```python
from build123d import *

# Parameters (mm, degrees)
F0_R     = 12.5
F1_DEPTH = 50
F2_SIZE  = 2
F3_R     = 8.107288
F4_DEPTH = 20
F5_W     = 25
F5_H     = 25
F6_DEPTH = 30
F7_SIZE  = 2.5
F8_R     = 10
F9_DEPTH = 50.001


with BuildPart() as f1:
    # F0 (on Top) → F1 (new body)
    with BuildSketch(Plane.XY):
        Circle(F0_R)
    extrude(amount=F1_DEPTH)

    # F2
    f2_edges = [f1.edges().sort_by_distance(p)[0] for p in [
        (-12.5, 0, 50),
        (-12.5, 0, 0),
    ]]
    chamfer(f2_edges, length=F2_SIZE)

    # F3 (on Front) → F4 (join)
    with BuildSketch(Plane.XZ):
        with Locations((0, 24.859188)):
            Circle(F3_R)
    extrude(amount=F4_DEPTH)

    # F5 (on face) → F6 (join)
    with BuildSketch(Plane.XZ.offset(20)):
        with Locations((0, 24.859188)):
            Rectangle(F5_W, F5_H)
    extrude(amount=F6_DEPTH)

    # F7
    f7_edges = [f1.edges().sort_by_distance(p)[0] for p in [
        (0, -50, 37.359188),
        (-12.5, -50, 24.859188),
        (0, -50, 12.359188),
        (12.5, -50, 24.859188),
    ]]
    chamfer(f7_edges, length=F7_SIZE)

    # F8 (on face) → F9 (cut, through all)
    with BuildSketch(Plane.XY.offset(50)):
        Circle(F8_R)
    extrude(amount=-F9_DEPTH, mode=Mode.SUBTRACT)


solid = f1.part
```
Could you check a few things on this model? Use its own coordinates, in mm. A direction names the side the tool comes from. Coordinates: 2 decimals unless noted, no trailing zeros. Order: outer loops, then holes, each group sorted by start corner. A loop starts at its lowest first (then second) coordinate and runs counter-clockwise, first axis right, second up. Notation, with made-up numbers: M 12,-23 L 30,-23 A19 ccw 30,0 Z; hole C 88,4 d1. An arc over 180 degrees is marked long. Use a Markdown table: item, result. Add a question column.
Q1. Which directions (+Z, -Z, +X, -X, +Y, -Y) give clear straight access to the entire face, cutting with the end or side of a thin tool? Please do faces 5 (the flat face through (-0.2, -20, 33.4)), 6 (the flat face through (0, -34, 37.359)), 7 (the flat face through (0, -34, 12.359)).
Q2. I'm going to push flat-ended pins straight in: pin 1 (7.5 mm diameter, centred on x = -4, y = -37, fed in from +Z); pin 2 (1.5 mm diameter, centred on x = -0.5, z = 40, fed in from -Y). Where does each tip first touch, or does it pass through?
Q3. I want a section at A-A on y = 0. List the corners of the cut face in (x, z) for me.
Q4. I want a section at D-D on y = -36. List the corners of the cut face in (x, z) for me, then the cut area to 3 significant figures.
Q5. We'd pull the mould along Y, two halves only. Please class faces 1 (the cylindrical face through (-2.17, -9.76, 25.35)), 2 (the cylindrical face through (-1.627, 12.394, 24.678)), 3 (the flat face through (-12.5, -34, 25)), 4 (the flat face through (11, -49, 25)): pulls with the +Y half, pulls with the -Y half, needs draft (parallel to the pull), parting line crosses it, or undercut.
Q6. I want a section at C-C on z = 31. List the corners of the cut face in (x, y) for me, then the cut area to 3 significant figures.
Q7. If I drill on L1, parallel to Y at x = 0, z = 26.5; L2, parallel to Y at x = 3.25, z = 13; L3, parallel to Y at x = 0, z = 36.5, over which ranges is the centre line in solid material (lowest first)?
Q8. I want a section at B-B on x = 0. List the corners of the cut face in (y, z) for me.
Checked values:
| question | item | result |
|---|---|---|
| 1 | face 5 | none |
| 1 | face 6 | +Z, +X, -X, -Y |
| 1 | face 7 | -Z, +X, -X, -Y |
| 2 | pin 1 | z = 37.36 |
| 2 | pin 2 | y = -12.5 |
| 3 | outline | M -12.5,2 L -10.5,0 L -10,0 L -10,50 L -10.5,50 L -12.5,48 Z; M 10,0 L 10.5,0 L 12.5,2 L 12.5,48 L 10.5,50 L 10,50 Z |
| 4 | outline | M -12.5,12.36 L 12.5,12.36 L 12.5,37.36 L -12.5,37.36 Z |
| 4 | area | 625 mm² |
| 5 | face 1 | undercut |
| 5 | face 2 | undercut |
| 5 | face 3 | needs draft |
| 5 | face 4 | pulls with the -Y half |
| 6 | outline | M -12.5,-47.5 L -10,-50 L 10,-50 L 12.5,-47.5 L 12.5,-20 L 5.29,-20 L 5.29,-11.32 A12.5 ccw long -5.29,-11.32 L -5.29,-20 L -12.5,-20 Z; hole C 0,0 d20 |
| 6 | area | 1,000 mm² |
| 7 | L1 | -50 to -10, 10 to 12.5 |
| 7 | L2 | -48.14 to -20, -12.07 to -9.46, 9.46 to 12.07 |
| 7 | L3 | -48.36 to -20, -12.5 to -10, 10 to 12.5 |
| 8 | outline | M -50,14.86 L -47.5,12.36 L -20,12.36 L -20,16.75 L -12.5,16.75 L -12.5,2 L -10.5,0 L -10,0 L -10,50 L -10.5,50 L -12.5,48 L -12.5,32.97 L -20,32.97 L -20,37.36 L -47.5,37.36 L -50,34.86 Z; M 10,0 L 10.5,0 L 12.5,2 L 12.5,48 L 10.5,50 L 10,50 Z |
